```python
from build123d import *

# Parameters (mm, degrees)
F1_DEPTH = 50.8
F3_D     = 33.02
F4_SIZE  = 7.62
F5_SIZE  = 7.62
F7_D     = 5.08
F9_D     = 6.35


with BuildPart() as f1:
    # F0 (on Front) → F1 (new body)
    with BuildSketch(Plane.XZ):
        Polygon((72.081462, 24.570465), (0, 0), (0, -23.26379), (72.081462, 0), align=None)
    extrude(amount=F1_DEPTH)

    # F3 (through all)
    with Locations(Plane(origin=(0, 0, 0), x_dir=(0.946521, 0, 0.322641), z_dir=(-0.322641, 0, 0.946521))):
        with Locations((38.495995, -25.001924)):
            Hole(F3_D / 2)

    # F4
    f4_edges = [f1.edges().sort_by_distance(p)[0] for p in [
        (36.040731, -50.8, -11.631895),
        (72.081462, -50.8, 12.285233),
        (36.040731, -50.8, 12.285233),
        (0, -50.8, -11.631895),
    ]]
    chamfer(f4_edges, length=F4_SIZE)

    # F5
    f5_edges = [f1.edges().sort_by_distance(p)[0] for p in [
        (36.040731, 0, -11.631895),
        (72.081462, 0, 12.285233),
        (36.040731, 0, 12.285233),
        (0, 0, -11.631895),
    ]]
    chamfer(f5_edges, length=F5_SIZE)

    # F7 (through all)
    with Locations(Plane(origin=(0, 0, 0), x_dir=(0.946521, 0, 0.322641), z_dir=(-0.322641, 0, 0.946521))):
        with Locations((65.759569, -26.372515)):
            Hole(F7_D / 2)

    # F9 (through all)
    with Locations(Plane(origin=(0, 0, 0), x_dir=(0.946521, 0, 0.322641), z_dir=(-0.322641, 0, 0.946521))):
        with Locations((11.439297, -25.4)):
            Hole(F9_D / 2)


solid = f1.part
```
Here's how the part is built. I have some questions about the finished solid (model axes, mm). Round coordinates to 2 decimals unless told otherwise and drop trailing zeros. Order: outer loops, then holes, each group sorted by start corner. A loop starts at its lowest first (then second) coordinate and runs counter-clockwise, first axis right, second up. Notation, with made-up numbers: M 15.25,-20.75 L 36.25,-20.75 A24 ccw 36.25,7.25 Z; hole C 49,61.25 d7. An arc over 180 degrees is marked long. Answer as CSV lines item,"result".
Item 1: We'd pull the mould along Y, two halves only. Please class faces 1 (the cylindrical face through (52.61, -35.05, 5.58)), 2 (the flat face through (34.382, -46.937, -8.22)), 3 (the flat face through (34.382, -3.863, -8.22)): +Y half, -Y half, draft (parallel to the pull), parting line (faces both ways), or undercut.
From the geometry:
face 1,"undercut"
face 2,"-Y half"
face 3,"+Y half"
Item 2: Imagine slicing it at B-B on x = 6. List the corners of the cut face in (y, z) for me, and give its area (3 significant figures).
From the geometry:
outline,"M -49.18,-15.02 L -43.18,-21.33 L -7.62,-21.33 L -1.62,-15.02 L -1.62,-4.29 L -7.62,2.05 L -43.18,2.05 L -49.18,-4.29 Z"
area,"1,040 mm2"
Item 3: Imagine slicing it at A-A on y = -38. List the corners of the cut face in (x, z) for me (3 decimals).
From the geometry:
outline,"M 0,-23.264 L 34.095,-12.26 L 26.802,9.136 L 0,0 Z; M 46.073,15.705 L 53.473,-6.006 L 72.081,0 L 72.081,24.57 Z"
Item 4: Imagine slicing it at D-D on y = -5. List the corners of the cut face in (x, z) for me.
From the geometry:
outline,"M 2.62,-19.67 L 69.46,1.91 L 69.46,20.91 L 2.62,-1.87 Z"
Item 5: For pin 1 (8 mm diameter, centred on x = 15.5, y = -6, fed in from +Z); pin 2 (1.5 mm diameter, centred on x = 61.5, y = -17.5, fed in from -Z); pin 3 (1 mm diameter, centred on x = 29, y = -25, fed in from -Z); pin 4 (3 mm diameter, centred on y = -37.5, z = 16.5, fed in from -X), each with a flat end and sliding along its axis, tell me the tip position at first contact or that it passes through.
From the geometry:
pin 1,"z = 6.53"
pin 2,"z = -3.66"
pin 3,"through"
pin 4,"x = 45.33"
Item 6: Please list where these lines run through material, in increasing order: L1, parallel to Y at x = 41, z = 10; L2, parallel to Y at x = 11.5, z = 2; L3, parallel to X at y = -27, z = -1. Write a range as [from, to].
From the geometry:
L1,"[-46.94, -41.13], [-8.88, -3.86]"
L2,"[-45, -28.57], [-22.23, -5.8]"
L3,"[0, 9.53], [15.32, 23.7], [58.33, 67.22]"
Item 7: Imagine slicing it at C-C on y = -12. List the corners of the cut face in (x, z) for me.
From the geometry:
outline,"M 0,-23.26 L 34.1,-12.26 L 26.81,9.14 L 0,0 Z; M 46.07,15.7 L 53.47,-6.01 L 72.08,0 L 72.08,24.57 Z"
